Check sheet for the modelled part. Datum: model origin and axes. Units: mm. Face numbers are marked on the shaded views. Round coordinates to 2 decimals unless told otherwise and drop trailing zeros. Write each loop counter-clockwise with the first axis right and the second up, starting at its lowest first coordinate (ties: lowest second). Pieces come first, ordered by that corner, then holes. Notation, with made-up numbers: (42, 83.25) -> (50, 83.25) arc R10 cw to (50, 100.25) -> close; hole circle Ø6 at (-21.5, 45.25). An arc over 180 degrees is marked (long way). One line per item, written item: value.
from build123d import *

# Parameters (mm, degrees)
F0_W     = 270
F0_H     = 270
F0_R     = 2.75
F0_R_2   = 2.25
F0_R_3   = 12.5
F1_DEPTH = 12.7
F2_R     = 3.75
F2_R_2   = 2.25
F3_DEPTH = 3.7
F4_R     = 12.5
F5_DEPTH = 7.7
F7_DEPTH = 12.7


with BuildPart() as f1:
    # F0 (on Top) → F1 (new body)
    with BuildSketch(Plane.XY):
        with Locations((135, 135)):
            Rectangle(F0_W, F0_H)
        with Locations((20, 20)):
            Circle(F0_R, mode=Mode.SUBTRACT)
        with Locations((66, 20)):
            Circle(F0_R_2, mode=Mode.SUBTRACT)
        with Locations((20, 66)):
            Circle(F0_R_2, mode=Mode.SUBTRACT)
        with Locations((112, 20)):
            Circle(F0_R_2, mode=Mode.SUBTRACT)
        with Locations((20, 112)):
            Circle(F0_R_2, mode=Mode.SUBTRACT)
        with Locations((158, 20)):
            Circle(F0_R_2, mode=Mode.SUBTRACT)
        with Locations((204, 20)):
            Circle(F0_R_2, mode=Mode.SUBTRACT)
        with Locations((250, 20)):
            Circle(F0_R, mode=Mode.SUBTRACT)
        with Locations((250, 66)):
            Circle(F0_R_2, mode=Mode.SUBTRACT)
        with Locations((250, 112)):
            Circle(F0_R_2, mode=Mode.SUBTRACT)
        with Locations((20, 158)):
            Circle(F0_R_2, mode=Mode.SUBTRACT)
        with Locations((20, 204)):
            Circle(F0_R_2, mode=Mode.SUBTRACT)
        with Locations((20, 250)):
            Circle(F0_R, mode=Mode.SUBTRACT)
        with Locations((66, 250)):
            Circle(F0_R_2, mode=Mode.SUBTRACT)
        with Locations((112, 250)):
            Circle(F0_R_2, mode=Mode.SUBTRACT)
        with Locations((135, 135)):
            Circle(F0_R_3, mode=Mode.SUBTRACT)
        with Locations((250, 158)):
            Circle(F0_R_2, mode=Mode.SUBTRACT)
        with Locations((158, 250)):
            Circle(F0_R_2, mode=Mode.SUBTRACT)
        with Locations((250, 204)):
            Circle(F0_R_2, mode=Mode.SUBTRACT)
        with Locations((204, 250)):
            Circle(F0_R_2, mode=Mode.SUBTRACT)
        with Locations((250, 250)):
            Circle(F0_R, mode=Mode.SUBTRACT)
    extrude(amount=F1_DEPTH)

    # F2 (on face) → F3 (cut)
    with BuildSketch(Plane.XY):
        with Locations((20, 204)):
            Circle(F2_R)
        with Locations((20, 204)):
            Circle(F2_R_2, mode=Mode.SUBTRACT)
        with Locations((66, 250)):
            Circle(F2_R)
        with Locations((66, 250)):
            Circle(F2_R_2, mode=Mode.SUBTRACT)
        with Locations((20, 158)):
            Circle(F2_R)
        with Locations((20, 158)):
            Circle(F2_R_2, mode=Mode.SUBTRACT)
        with Locations((20, 112)):
            Circle(F2_R)
        with Locations((20, 112)):
            Circle(F2_R_2, mode=Mode.SUBTRACT)
        with Locations((20, 66)):
            Circle(F2_R)
        with Locations((20, 66)):
            Circle(F2_R_2, mode=Mode.SUBTRACT)
        with Locations((66, 20)):
            Circle(F2_R)
        with Locations((66, 20)):
            Circle(F2_R_2, mode=Mode.SUBTRACT)
        with Locations((112, 20)):
            Circle(F2_R)
        with Locations((112, 20)):
            Circle(F2_R_2, mode=Mode.SUBTRACT)
        with Locations((158, 20)):
            Circle(F2_R)
        with Locations((158, 20)):
            Circle(F2_R_2, mode=Mode.SUBTRACT)
        with Locations((204, 20)):
            Circle(F2_R)
        with Locations((204, 20)):
            Circle(F2_R_2, mode=Mode.SUBTRACT)
        with Locations((250, 66)):
            Circle(F2_R)
        with Locations((250, 66)):
            Circle(F2_R_2, mode=Mode.SUBTRACT)
        with Locations((250, 112)):
            Circle(F2_R)
        with Locations((250, 112)):
            Circle(F2_R_2, mode=Mode.SUBTRACT)
        with Locations((250, 158)):
            Circle(F2_R)
        with Locations((250, 158)):
            Circle(F2_R_2, mode=Mode.SUBTRACT)
        with Locations((250, 204)):
            Circle(F2_R)
        with Locations((250, 204)):
            Circle(F2_R_2, mode=Mode.SUBTRACT)
        with Locations((112, 250)):
            Circle(F2_R)
        with Locations((112, 250)):
            Circle(F2_R_2, mode=Mode.SUBTRACT)
        with Locations((158, 250)):
            Circle(F2_R)
        with Locations((158, 250)):
            Circle(F2_R_2, mode=Mode.SUBTRACT)
        with Locations((204, 250)):
            Circle(F2_R)
        with Locations((204, 250)):
            Circle(F2_R_2, mode=Mode.SUBTRACT)
    extrude(amount=F3_DEPTH, mode=Mode.SUBTRACT)

    # F4 (on face) → F5 (cut)
    with BuildSketch(Plane.XY.offset(12.7)):
        with BuildLine():
            Line((220, 240), (50, 240))
            ThreePointArc((50, 240), (35.857864, 234.142136), (30, 220))
            Line((30, 220), (30, 50))
            ThreePointArc((30, 50), (35.857864, 35.857864), (50, 30))
            Line((50, 30), (220, 30))
            ThreePointArc((220, 30), (234.142136, 35.857864), (240, 50))
            Line((240, 50), (240, 220))
            ThreePointArc((240, 220), (234.142136, 234.142136), (220, 240))
        make_face()
        with Locations((135, 135)):
            Circle(F4_R, mode=Mode.SUBTRACT)
    extrude(amount=-F5_DEPTH, mode=Mode.SUBTRACT)

    # F6 (on face) → F7 (join)
    with BuildSketch(Plane.XY):
        with BuildLine():
            Line((87.5, 170.5), (82.5, 170.5))
            Line((82.5, 170.5), (82.5, 142.5))
            ThreePointArc((82.5, 142.5), (81.035534, 138.964466), (77.5, 137.5))
            Line((77.5, 137.5), (49.5, 137.5))
            Line((49.5, 137.5), (49.5, 132.5))
            Line((49.5, 132.5), (77.5, 132.5))
            ThreePointArc((77.5, 132.5), (81.035534, 131.035534), (82.5, 127.5))
            Line((82.5, 127.5), (82.5, 99.5))
            Line((82.5, 99.5), (87.5, 99.5))
            Line((87.5, 99.5), (87.5, 127.5))
            ThreePointArc((87.5, 127.5), (88.964466, 131.035534), (92.5, 132.5))
            Line((92.5, 132.5), (120.5, 132.5))
            Line((120.5, 132.5), (120.5, 137.5))
            Line((120.5, 137.5), (92.5, 137.5))
            ThreePointArc((92.5, 137.5), (88.964466, 138.964466), (87.5, 142.5))
            Line((87.5, 142.5), (87.5, 170.5))
        make_face()
        with BuildLine():
            Line((182.5, 170.5), (182.5, 142.5))
            ThreePointArc((182.5, 142.5), (181.035534, 138.964466), (177.5, 137.5))
            Line((177.5, 137.5), (149.5, 137.5))
            Line((149.5, 137.5), (149.5, 132.5))
            Line((149.5, 132.5), (177.5, 132.5))
            ThreePointArc((177.5, 132.5), (181.035534, 131.035534), (182.5, 127.5))
            Line((182.5, 127.5), (182.5, 99.5))
            Line((182.5, 99.5), (187.5, 99.5))
            Line((187.5, 99.5), (187.5, 127.5))
            ThreePointArc((187.5, 127.5), (188.964466, 131.035534), (192.5, 132.5))
            Line((192.5, 132.5), (220.5, 132.5))
            Line((220.5, 132.5), (220.5, 137.5))
            Line((220.5, 137.5), (192.5, 137.5))
            ThreePointArc((192.5, 137.5), (188.964466, 138.964466), (187.5, 142.5))
            Line((187.5, 142.5), (187.5, 170.5))
            Line((187.5, 170.5), (182.5, 170.5))
        make_face()
        with BuildLine():
            Line((137.5, 192.5), (137.5, 220.5))
            Line((137.5, 220.5), (132.5, 220.5))
            Line((132.5, 220.5), (132.5, 192.5))
            ThreePointArc((132.5, 192.5), (131.035534, 188.964466), (127.5, 187.5))
            Line((127.5, 187.5), (99.5, 187.5))
            Line((99.5, 187.5), (99.5, 182.5))
            Line((99.5, 182.5), (127.5, 182.5))
            ThreePointArc((127.5, 182.5), (131.035534, 181.035534), (132.5, 177.5))
            Line((132.5, 177.5), (132.5, 149.5))
            Line((132.5, 149.5), (137.5, 149.5))
            Line((137.5, 149.5), (137.5, 177.5))
            ThreePointArc((137.5, 177.5), (138.964466, 181.035534), (142.5, 182.5))
            Line((142.5, 182.5), (170.5, 182.5))
            Line((170.5, 182.5), (170.5, 187.5))
            Line((170.5, 187.5), (142.5, 187.5))
            ThreePointArc((142.5, 187.5), (138.964466, 188.964466), (137.5, 192.5))
        make_face()
        with BuildLine():
            Line((132.5, 77.5), (132.5, 49.5))
            Line((132.5, 49.5), (137.5, 49.5))
            Line((137.5, 49.5), (137.5, 77.5))
            ThreePointArc((137.5, 77.5), (138.964466, 81.035534), (142.5, 82.5))
            Line((142.5, 82.5), (170.5, 82.5))
            Line((170.5, 82.5), (170.5, 87.5))
            Line((170.5, 87.5), (142.5, 87.5))
            ThreePointArc((142.5, 87.5), (138.964466, 88.964466), (137.5, 92.5))
            Line((137.5, 92.5), (137.5, 120.5))
            Line((137.5, 120.5), (132.5, 120.5))
            Line((132.5, 120.5), (132.5, 92.5))
            ThreePointArc((132.5, 92.5), (131.035534, 88.964466), (127.5, 87.5))
            Line((127.5, 87.5), (99.5, 87.5))
            Line((99.5, 87.5), (99.5, 82.5))
            Line((99.5, 82.5), (127.5, 82.5))
            ThreePointArc((127.5, 82.5), (131.035534, 81.035534), (132.5, 77.5))
        make_face()
    extrude(amount=F7_DEPTH)


solid = f1.part
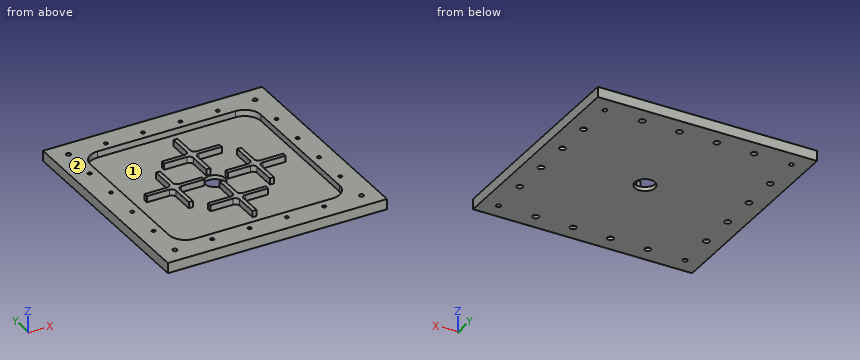
Item 1: Sectioned sample at A-A (x = 214.5). Enter the section's corners in (y, z), then the cut area to 3 significant figures.
Result set:
outline: (0, 0) -> (270, 0) -> (270, 12.7) -> (240, 12.7) -> (240, 5) -> (137.5, 5) -> (137.5, 12.7) -> (132.5, 12.7) -> (132.5, 5) -> (30, 5) -> (30, 12.7) -> (0, 12.7) -> close
area: 1,850 mm^2
Item 2: Material ranges on line 1 along Y through (x, z) = (127.5, 10.25); line 2 along Y through (x, z) = (163, 11); line 3 along Y through (x, z) = (158, 1.6), recorded low to high.
Result set:
line 1: 0 to 30, 82.5 to 87.5, 182.5 to 187.5, 240 to 270
line 2: 0 to 30, 82.5 to 87.5, 132.5 to 137.5, 182.5 to 187.5, 240 to 270
line 3: 0 to 16.25, 23.75 to 246.25, 253.75 to 270
Item 3: Release check for a two-part mould opening along Y. For the marked faces 1 and 2 record: pulls with the +Y half, pulls with the -Y half, needs draft (parallel to the pull), parting line crosses it, or undercut.
Result set:
face 1: undercut
face 2: needs draft
Item 4: Depth check by flat-ended pin: pin 1 (5 mm diameter, centred on x = 228, y = 160.5, fed in from +Z); pin 2 (2 mm diameter, centred on x = 21, y = 65, fed in from -Z). Enter the tip coordinate at first touch or a pass-through.
Result set:
pin 1: z = 5
pin 2: z = 3.7
Item 5: Sectioned sample at B-B (z = 8.75). State how many separate pieces and enclosed holes the cut face has, then the cut area to 3 significant figures.
Result set:
separate pieces: 5
enclosed holes: 21
area: 31,600 mm^2
